from build123d import *

# Parameters (mm, degrees)
SKETCH1_W           = 60
SKETCH1_H           = 35
BOSS_EXTRUDE1_DEPTH = 8
SKETCH2_W           = 15
SKETCH2_H           = 6
BOSS_EXTRUDE2_DEPTH = 20
SKETCH3_W           = 20
SKETCH3_H           = 15
CUT_EXTRUDE2_DEPTH  = 41.078048855


with BuildPart() as part:
    # Sketch1 → Boss-Extrude1 (new body)
    with BuildSketch(Plane(origin=(0, 0, 0), x_dir=(1, 0, 0), z_dir=(0, 1, 0))):
        Rectangle(SKETCH1_W, SKETCH1_H)
    extrude(amount=BOSS_EXTRUDE1_DEPTH)

    # Sketch2 → Boss-Extrude2 (add)
    with BuildSketch(Plane(origin=(0, 0, 0), x_dir=(1, 0, 0), z_dir=(0, 1, 0))):
        with Locations((-22.5, 14.5)):
            Rectangle(SKETCH2_W, SKETCH2_H)
        with Locations((22.5, -14.5)):
            Rectangle(SKETCH2_W, SKETCH2_H)
    extrude(amount=BOSS_EXTRUDE2_DEPTH)

    # Sketch3 → Cut-Extrude2 (cut, through all)
    with BuildSketch(Plane(origin=(0, 0, 0), x_dir=(1, 0, 0), z_dir=(0, 1, 0))):
        Rectangle(SKETCH3_W, SKETCH3_H)
    extrude(amount=CUT_EXTRUDE2_DEPTH, mode=Mode.SUBTRACT)


solid = part.part
The listing builds one solid part. Answer for the finished solid, in the listing's coordinates (mm). A direction names the side the tool comes from. Give positions to 0.01 mm unless a question says otherwise; leave off trailing zeros. Loops run counter-clockwise (first coordinate to the right, second up) from the corner with the lowest first, then second, coordinate; pieces in that order, holes last. Notation, with made-up numbers: (-19.5, 32.5) - (-1.5, 32.5) arc R31 cw to (-1.5, 56.5) - close; hole circle Ø7 at (40.25, 16). An arc over 180 degrees is marked (long way). Use one line per item in the form item = value.
1. Given pin 1 Ø5 at (y, z) = (16.5, 14.5) entering from -X; pin 2 Ø10 at (x, z) = (2, 1.5) entering from +Y; pin 3 Ø6.5 at (y, z) = (14.5, -14.5) entering from +X, each flat-ended and moving along its own axis, determine where each tip first touches the part or whether it passes through.
Calculated:
pin_1 = 15
pin_2 = through
pin_3 = -15
2. Section C-C on y = 3.25 is taken. Give the vertices of the cut face in (x, z).
Calculated:
outline = (-30, -17.5) - (30, -17.5) - (30, 17.5) - (-30, 17.5) - close; hole (-10, -7.5) - (10, -7.5) - (10, 7.5) - (-10, 7.5) - close
3. Section A-A on x = -8 is taken. Give the vertices of the cut face in (y, z), then the cut area to 3 significant figures.
Calculated:
outline = (0, -17.5) - (8, -17.5) - (8, -7.5) - (0, -7.5) - close; (0, 7.5) - (8, 7.5) - (8, 17.5) - (0, 17.5) - close
area = 160 mm^2
4. Find the intervals of material crossed by line 1 along Y through (x, z) = (-18, -5); line 2 along Z through (x, y) = (26.5, 15.5); line 3 along X through (y, z) = (11.75, 13), in increasing order. Write a range as [from, to].
Calculated:
line_1 = [0, 8]
line_2 = [11.5, 17.5]
line_3 = [15, 30]
5. Section B-B on y = 14.75 is taken. Give the vertices of the cut face in (x, z), then the cut area to 3 significant figures.
Calculated:
outline = (-30, -17.5) - (-15, -17.5) - (-15, -11.5) - (-30, -11.5) - close; (15, 11.5) - (30, 11.5) - (30, 17.5) - (15, 17.5) - close
area = 180 mm^2
6. Which of the six approach directions +Z, -Z, +X, -X, +Y, -Y give full straight-line access (tool end or side, diameter ignored) to faces 1 (the face through (30, 5, 4)), 2 (the face through (-10, 4, 0)), 3 (the face through (15, 14, 15)), 4 (the face through (-23, 14, -11.5)), 5 (the face through (-30, 5, 0))?
Calculated:
face_1 = +Z, -Z, +X, +Y, -Y
face_2 = +Y, -Y
face_3 = +Z, -Z, -X, +Y
face_4 = +Z, +X, -X, +Y
face_5 = +Z, -Z, -X, +Y, -Y
7. Section D-D on z = 13 is taken. Give the vertices of the cut face in (x, y).
Calculated:
outline = (-30, 0) - (30, 0) - (30, 20) - (15, 20) - (15, 8) - (-30, 8) - close
8. The mould has two halves that part along Z. Classify faces 6 (the face through (22, 14, 11.5)), 7 (the face through (-15, 14, -14)), 8 (the face through (10, 4, 0)): pulls with the +Z half, pulls with the -Z half, needs draft (parallel to the pull), parting line crosses it, or undercut.
Calculated:
face_6 = pulls with the -Z half
face_7 = needs draft
face_8 = undercut
